The drawing under review shows one solid part. Ordinate dimensions are in mm from its lowest x, y, z. A direction names the side the tool comes from. Round coordinates to 2 decimals unless told otherwise and drop trailing zeros. Order: outer loops, then holes, each group sorted by start corner. A loop starts at its lowest first (then second) coordinate and runs counter-clockwise, first axis right, second up. Notation, with made-up numbers: M 21.25,-17.5 L 63.25,-17.5 A19 ccw 63.25,-8.5 Z; hole C -13,59 d4. An arc over 180 degrees is marked long. Answer as a JSON object with one key per item and string values.
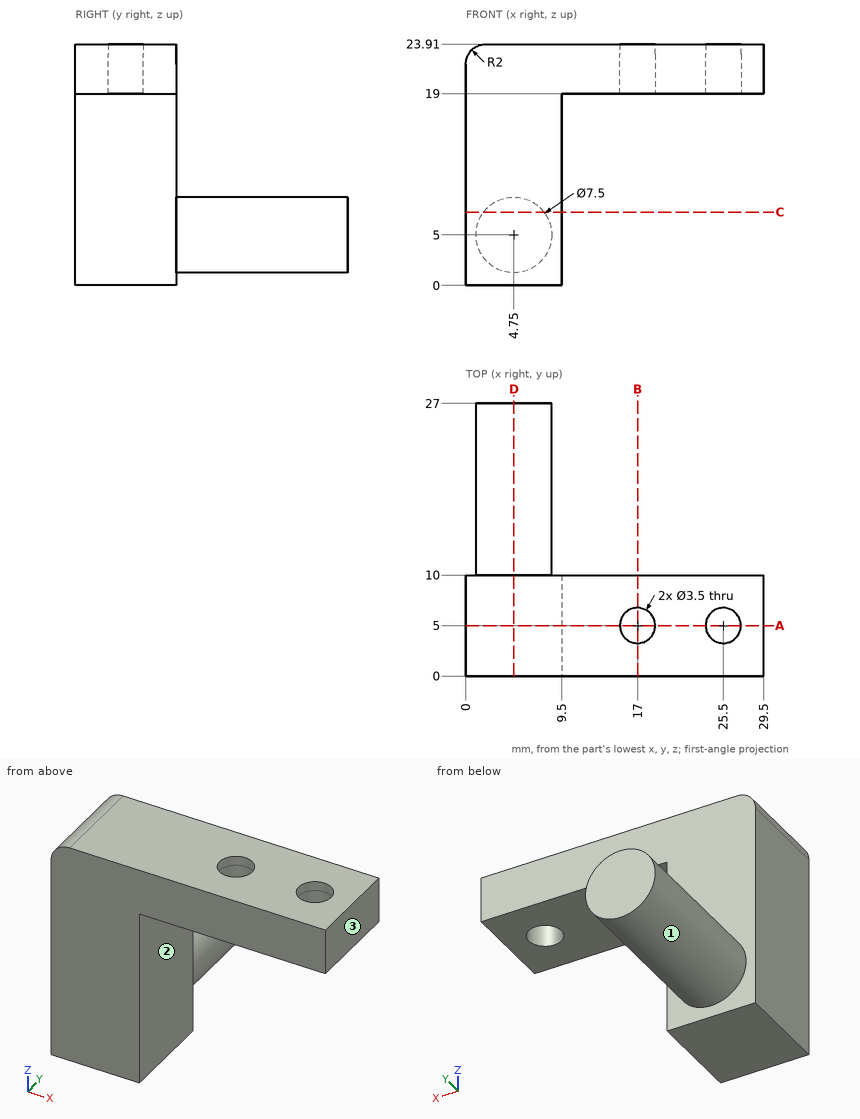
1) Add section D-D on x = 4.75. State the section outline as (y, z) points.
Geometry check:
{"outline": "M 0,0 L 10,0 L 10,1.25 L 27,1.25 L 27,8.75 L 10,8.75 L 10,23.91 L 0,23.91 Z"}
2) Add section B-B on x = 17. State the section outline as (y, z) points.
Geometry check:
{"outline": "M 0,19 L 3.25,19 L 3.25,23.91 L 0,23.91 Z; M 6.75,19 L 10,19 L 10,23.91 L 6.75,23.91 Z"}
3) Add section A-A on y = 5. State the section outline as (x, z) points.
Geometry check:
{"outline": "M 0,0 L 9.5,0 L 9.5,19 L 15.25,19 L 15.25,23.91 L 2,23.91 A2 ccw 0,21.91 Z; M 18.75,19 L 23.75,19 L 23.75,23.91 L 18.75,23.91 Z; M 27.25,19 L 29.5,19 L 29.5,23.91 L 27.25,23.91 Z"}
4) For L1, parallel to Y at x = 25.5, z = 23.7; L2, parallel to Y at x = 13, z = 22; L3, parallel to Z at x = 18.75, y = 6.75, list the stretches that pass through material, from the lowest coordinate up.
Geometry check:
{"L1": "y = 0 to 3.25, 6.75 to 10", "L2": "y = 0 to 10", "L3": "z = 19 to 23.91"}
5) Insertion check: P1, Ø1, axis at x = 11.5, z = 9, coming from the +Y side; P2, Ø3, axis at x = 16, y = 6.5, coming from the -Z side; P3, Ø1.5, axis at x = 7, z = 20, coming from the -Y side; P4, Ø12, axis at x = 15.5, z = 17, coming from the +Y side. Each pin has a flat end and moves straight along its axis. Give the tip position at first contact, or say it passes through.
Geometry check:
{"P1": "passes through", "P2": "stops at z = 19", "P3": "stops at y = 0", "P4": "stops at y = 10"}
6) Add section C-C on z = 7.25. State the section outline as (x, y) points.
Geometry check:
{"outline": "M 0,0 L 9.5,0 L 9.5,10 L 7.75,10 L 7.75,27 L 1.75,27 L 1.75,10 L 0,10 Z"}
7) Machinability: for the marked faces 1, 2 and 3, which of the approach directions +Z, -Z, +X, -X, +Y, -Y give a long, thin tool a straight path to every point of the face, cutting with its end or side? Answer none if there is none.
Geometry check:
{"face 1": "+Y", "face 2": "-Z, +X, +Y, -Y", "face 3": "+Z, -Z, +X, +Y, -Y"}
